Read the model definition and answer for the solid it produces. Units are mm, in the model's axes. Face numbers are marked on the shaded views. A direction names the side the tool comes from. Coordinates: 2 decimals unless noted, no trailing zeros. Loops run counter-clockwise (first coordinate to the right, second up) from the corner with the lowest first, then second, coordinate; pieces in that order, holes last. Notation, with made-up numbers: (72.5, 19.5) -> (102.5, 19.5) arc R25 ccw to (102.5, 56.5) -> close; hole circle Ø3 at (64.25, -29). An arc over 180 degrees is marked (long way). Answer as a JSON object with one key per item and string values. Group by question number.
Q1. Straight lines are drawn through the part: line 1 along Y through (x, z) = (0, 5.2); line 2 along Z through (x, y) = (1.25, 13.5); line 3 along Z through (x, y) = (1, 13.75). For each, find the intervals that lie inside material, in ascending order. Write a range as [from, to].
Q2. Determine the mould class of the marked faces 3, 4 and 5 for opening direction Y: released by +Y, released by -Y, zero draft, split by the parting line, or undercut.
Q3. The part is cut by section D-D on x = 10.25. Write down the section's boundary in (y, z), and give its area (3 significant figures).
Q4. For the marked faces 1 and 2, determine the directions among +Z, -Z, +X, -X, +Y, -Y from which every point of the face is accessible in a straight line to the end or side of a thin tool.
Q5. Each of these flat-tipped pins is pushed along its axis until it touches: P1, Ø8, axis at x = 8.5, z = -4, coming from the -Y side; P2, Ø2, axis at x = -10.5, y = 14, coming from the +Z side; P3, Ø2.5, axis at x = -9.09, z = 5.25, coming from the +Y side; P4, Ø8, axis at y = 3.5, z = -9.5, coming from the +X side. Where does it stop, or does it pass through?
Q6. The part is cut by section B-B on x = 0. Write down the section's boundary in (y, z), and give its area (3 significant figures).
Q7. The part is cut by section A-A on z = 5.25. Write down the section's boundary in (x, y), and give its area (3 significant figures).
Q8. The part is cut by section C-C on z = 0. Write down the section's boundary in (x, y), and give its area (3 significant figures).
from build123d import *

# Parameters (mm, degrees)
ESQUISSE2_R             = 1.5
ENL_V_MAT_EXTRU_1_DEPTH = 26.455844123
ESQUISSE3_R             = 2
ENL_V_MAT_EXTRU_2_DEPTH = 26.455844123


with BuildPart() as part:
    # Esquisse1 → Révolution1 (revolve)
    with BuildSketch(Plane.XY, mode=Mode.PRIVATE) as r_volution1_sk:
        Polygon((-3, 0), (-3, 16), (-14, 16), (-14, 12), (-7.5, 12), (-7.5, 0), align=None)
    revolve(r_volution1_sk.sketch.rotate(Axis((0, 0, 0), (0, 1, 0)), 270), axis=Axis((0, 0, 0), (0, 1, 0)))

    # Esquisse2 → Enlèv. mat.-Extru.1 (cut, through all)
    with BuildSketch(Plane(origin=(0, 16, 0), x_dir=(1, 0, 0), z_dir=(0, 1, 0))):
        with Locations(Location((9.09326674, -5.25, 0), (0, 0, 270))):
            Circle(ESQUISSE2_R)
        with Locations(Location((-9.09326674, -5.25, 0), (0, 0, 270))):
            Circle(ESQUISSE2_R)
        with Locations(Location((0, 10.5, 0), (0, 0, 270))):
            Circle(ESQUISSE2_R)
    extrude(amount=-ENL_V_MAT_EXTRU_1_DEPTH, mode=Mode.SUBTRACT)

    # Esquisse3 → Enlèv. mat.-Extru.2 (cut, through all)
    with BuildSketch(Plane.XY):
        with Locations(Location((0, 8, 0), (0, 0, 180))):
            Circle(ESQUISSE3_R)
    extrude(amount=ENL_V_MAT_EXTRU_2_DEPTH, mode=Mode.SUBTRACT)


solid = part.part
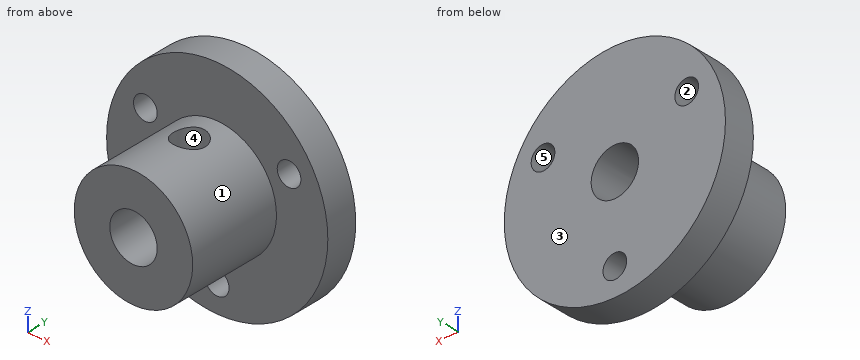
Final values:
{
 "1": {"line 1": "y = [0, 6], [10, 16]", "line 2": "z = [-13.94, -11.33], [-9.67, -2.73], [2.73, 13.94]", "line 3": "z = [-13.96, -11.62], [-9.38, -2.83], [2.83, 13.96]"},
 "2": {"face 3": "released by +Y", "face 4": "undercut", "face 5": "zero draft"},
 "3": {"outline": "(12, -9.54) -> (16, -9.54) -> (16, 4.3) -> (12, 4.3) -> close; (12, 6.2) -> (16, 6.2) -> (16, 9.54) -> (12, 9.54) -> close", "area": "68.6 mm2"},
 "4": {"face 1": "-Y", "face 2": "+Y, -Y"},
 "5": {"P1": "stops at y = 0", "P2": "stops at z = 10.28", "P3": "passes through", "P4": "stops at x = 5.1"},
 "6": {"outline": "(0, -7.5) -> (12, -7.5) -> (12, -9) -> (16, -9) -> (16, -3) -> (0, -3) -> close; (0, 3) -> (6, 3) -> (6, 7.5) -> (0, 7.5) -> close; (10, 3) -> (16, 3) -> (16, 14) -> (12, 14) -> (12, 7.5) -> (10, 7.5) -> close; (12, -14) -> (16, -14) -> (16, -12) -> (12, -12) -> close", "area": "166 mm2"},
 "7": {"outline": "(-12.98, 12) -> (-10.59, 12) -> (-10.59, 16) -> (-12.98, 16) -> close; (-7.59, 12) -> (-5.36, 12) -> (-5.36, 0) -> (5.36, 0) -> (5.36, 12) -> (7.59, 12) -> (7.59, 16) -> (-7.59, 16) -> close; (10.59, 12) -> (12.98, 12) -> (12.98, 16) -> (10.59, 16) -> close; hole circle Ø4 at (0, 8)", "area": "196 mm2"},
 "8": {"outline": "(-14, 12) -> (-7.5, 12) -> (-7.5, 0) -> (-3, 0) -> (-3, 16) -> (-14, 16) -> close; (3, 0) -> (7.5, 0) -> (7.5, 12) -> (14, 12) -> (14, 16) -> (3, 16) -> close", "area": "196 mm2"}
}
